The listing builds one solid part. Answer for the finished solid, in the listing's coordinates (mm). Coordinates: 2 decimals unless noted, no trailing zeros. Order: outer loops, then holes, each group sorted by start corner. A loop starts at its lowest first (then second) coordinate and runs counter-clockwise, first axis right, second up. Notation, with made-up numbers: (-22, 55.5) -> (21, 55.5) arc R16 cw to (21, 86.5) -> close; hole circle Ø2 at (-40, 69). An arc over 180 degrees is marked (long way). Write item = value, one per line. Start each with the question number.
```python
from build123d import *

# Parameters (mm, degrees)
REVOLVE_1_OUTLINE_R   = 10
REVOLVE_1_DEPTH       = 2
REVOLVE_START         = 2
REVOLVE_1_2_OUTLINE_R = 2.5
REVOLVE_1_2_DEPTH     = 1.5
SKETCH_2_R            = 1
SKETCH_2_R_2          = 0.5
CUT_EXTRUDE_2_DEPTH   = 15.282856857


# Read off the part's stored shape, not the designer's step: 旋转1
with BuildPart() as part:
    # 旋转1 outline → 旋转1 (new body)
    with BuildSketch(Plane(origin=(0, 0, 0), x_dir=(1, 0, 0), z_dir=(0, 1, 0))):
        Circle(REVOLVE_1_OUTLINE_R)
    extrude(amount=REVOLVE_1_DEPTH)

    # Revolve 1 2 outline → Revolve 1 2 (add)
    with BuildSketch(Plane(origin=(0, 0, 0), x_dir=(1, 0, 0), z_dir=(0, 1, 0)).offset(REVOLVE_START)):
        Circle(REVOLVE_1_2_OUTLINE_R)
    extrude(amount=REVOLVE_1_2_DEPTH)

    # 草图2 → 切除-拉伸2 (cut, through all)
    with BuildSketch(Plane(origin=(0, 2, 0), x_dir=(1, 0, 0), z_dir=(0, 1, 0))):
        with Locations(Location((-8, 0, 0), (0, 0, 180))):
            Circle(SKETCH_2_R)
        with Locations((4, 0)):
            Circle(SKETCH_2_R_2)
        with Locations((8, 0)):
            Circle(SKETCH_2_R)
        with Locations(Location((-4, 0, 0), (0, 0, 180))):
            Circle(SKETCH_2_R_2)
        with Locations(Location((0, 8, 0), (0, 0, 180))):
            Circle(SKETCH_2_R)
        with Locations((0, -8)):
            Circle(SKETCH_2_R)
    extrude(amount=-CUT_EXTRUDE_2_DEPTH, mode=Mode.SUBTRACT)


solid = part.part
```
Item 1: Section C-C, the plane z = 8 is taken. Give the vertices of the cut face in (x, y).
Item 2: Each of these flat-tipped pins is pushed along its axis until it touches: pin 1 (2.5 mm diameter, centred on x = 8, z = 0, fed in from -Y); pin 2 (1.5 mm diameter, centred on x = 3.5, y = 1.5, fed in from -Z); pin 3 (1.8 mm diameter, centred on x = 0, z = -8, fed in from +Y); pin 4 (3 mm diameter, centred on x = -4.5, z = -6.5, fed in from +Y). Where does it stop, or does it pass through?
Item 3: Section A-A, the plane z = 0 is taken. Give the vertices of the cut face in (x, y), then the cut area to 3 significant figures.
Item 4: For a pull along Z with two mould halves and no side action, classify faces 1 (the flat face through (2, 2, 2)), 2 (the cylindrical face through (-0.54, 2.74, 2.44)), 3 (the cylindrical face through (0, 1, -7)) as pulls with the +Z half, pulls with the -Z half, needs draft (parallel to the pull), parting line crosses it, or undercut.
Item 5: Consider probe 1 along Z at (x, y) = (0.25, 0.2); probe 2 along Z at (x, y) = (-4, 0.95); probe 3 along Y at (x, z) = (-3, 0). Determine where each line is inside the solid, lowest interval first.
Item 6: Section B-B, the plane x = -8 is taken. Give the vertices of the cut face in (y, z).
Item 7: Section D-D, the plane y = 1.15 is taken. Give the vertices of the cut face in (x, z), then the cut area to 3 significant figures.
A:
q1.outline = (-6, 0) -> (-1, 0) -> (-1, 2) -> (-6, 2) -> close; (1, 0) -> (6, 0) -> (6, 2) -> (1, 2) -> close
q2.pin_1 = 0
q2.pin_2 = -9.61
q2.pin_3 = through
q2.pin_4 = 2
q3.outline = (-10, 0) -> (-9, 0) -> (-9, 2) -> (-10, 2) -> close; (-7, 0) -> (-4.5, 0) -> (-4.5, 2) -> (-7, 2) -> close; (-3.5, 0) -> (3.5, 0) -> (3.5, 2) -> (2.5, 2) -> (2.5, 3.5) -> (-2.5, 3.5) -> (-2.5, 2) -> (-3.5, 2) -> close; (4.5, 0) -> (7, 0) -> (7, 2) -> (4.5, 2) -> close; (9, 0) -> (10, 0) -> (10, 2) -> (9, 2) -> close
q3.area = 35.5 mm^2
q4.face_1 = needs draft
q4.face_2 = parting line crosses it
q4.face_3 = undercut
q5.probe_1 = -10 to -8.97, -7.03 to 7.03, 8.97 to 10
q5.probe_2 = -9.17 to -0.5, 0.5 to 9.17
q5.probe_3 = 0 to 2
q6.outline = (0, -6) -> (2, -6) -> (2, -1) -> (0, -1) -> close; (0, 1) -> (2, 1) -> (2, 6) -> (0, 6) -> close
q7.outline = circle Ø20 at (0, 0); hole circle Ø2 at (-8, 0); hole circle Ø1 at (-4, 0); hole circle Ø2 at (0, -8); hole circle Ø2 at (0, 8); hole circle Ø1 at (4, 0); hole circle Ø2 at (8, 0)
q7.area = 300 mm^2
